Could you check a few things on this model? Use its own coordinates, in mm. Face numbers are marked on the shaded views. Round coordinates to 2 decimals unless told otherwise and drop trailing zeros. Write each loop counter-clockwise with the first axis right and the second up, starting at its lowest first coordinate (ties: lowest second). Pieces come first, ordered by that corner, then holes. Notation, with made-up numbers: (-21, 27) -> (-13, 27) arc R27 cw to (-13, 60) -> close; hole circle Ø9 at (41, 13). An arc over 180 degrees is marked (long way). One line per question, with ' | ' between items. Start each with the question number.
1. If I drill on line 1 along Y through (x, z) = (-1, 4.5); line 2 along Y through (x, z) = (3.5, 4.3); line 3 along Z through (x, y) = (2.25, 1.75), over which ranges is the centre line in solid material (lowest first)? Write a range as [from, to].
2. Imagine slicing it at B-B, the plane z = 4.75. List the corners of the cut face in (x, y) for me, and give its area (3 significant figures).
3. Imagine slicing it at C-C, the plane x = -1.5. List the corners of the cut face in (y, z) for me, and give its area (3 significant figures).
4. Thinking about a two-plate mould opening in Z: for the marked faces 1, 2 and 3, which applies, released by +Z, released by -Z, zero draft, split by the parting line, or undercut?
5. Imagine slicing it at D-D, the plane y = 5. List the corners of the cut face in (x, z) for me, and give its area (3 significant figures).
6. For pin 1 Ø2 at (x, z) = (-3.5, 4.5) entering from +Y, with a flat end and sliding along its axis, tell me the tip position at first contact or that it passes through.
7. Imagine slicing it at A-A, the plane y = 3. List the corners of the cut face in (x, z) for me.
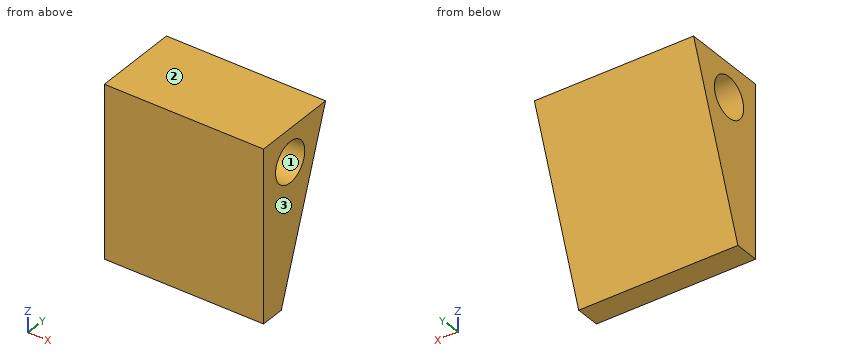
from build123d import *

# Parameters (mm, degrees)
SKETCH1_W           = 13
SKETCH1_H           = 14
BOSS_EXTRUDE1_DEPTH = 2
BOSS_EXTRUDE2_DEPTH = 13
SKETCH3_R           = 1.65
CUT_EXTRUDE1_DEPTH  = 13


with BuildPart() as part:
    # Sketch1 → Boss-Extrude1 (new body)
    with BuildSketch(Plane(origin=(0, 0, 0), x_dir=(1, 0, 0), z_dir=(0, 1, 0))):
        Rectangle(SKETCH1_W, SKETCH1_H)
    extrude(amount=BOSS_EXTRUDE1_DEPTH)

    # Sketch2 → Boss-Extrude2 (add)
    with BuildSketch(Plane(origin=(6.5, 0, 0), x_dir=(0, 0, -1), z_dir=(1, 0, 0))):
        Polygon((-7, 2), (-7, 7), (7, 2), align=None)
    extrude(amount=-BOSS_EXTRUDE2_DEPTH)

    # Sketch3 → Cut-Extrude1 (cut)
    with BuildSketch(Plane.ZY.offset(6.5)):
        with Locations((4.3, 3)):
            Circle(SKETCH3_R)
    extrude(amount=-CUT_EXTRUDE1_DEPTH, mode=Mode.SUBTRACT)


solid = part.part
Geometry results:
1) line 1: y = [0, 1.36], [4.64, 6.11] | line 2: y = [0, 1.35], [4.65, 6.04] | line 3: z = [-7, 3.22], [5.38, 7]
2) outline: (-6.5, 0) -> (6.5, 0) -> (6.5, 1.41) -> (-6.5, 1.41) -> close; (-6.5, 4.59) -> (6.5, 4.59) -> (6.5, 6.2) -> (-6.5, 6.2) -> close | area: 39.3 mm2
3) outline: (0, -7) -> (2, -7) -> (7, 7) -> (0, 7) -> close; hole circle Ø3.3 at (3, 4.3) | area: 54.4 mm2
4) face 1: undercut | face 2: released by +Z | face 3: zero draft
5) outline: (-6.5, 1.4) -> (6.5, 1.4) -> (6.5, 7) -> (-6.5, 7) -> close | area: 72.8 mm2
6) pin 1: stops at y = 6.46
7) outline: (-6.5, -4.2) -> (6.5, -4.2) -> (6.5, 2.65) -> (-6.5, 2.65) -> close; (-6.5, 5.95) -> (6.5, 5.95) -> (6.5, 7) -> (-6.5, 7) -> close
